```python
from build123d import *

# Parameters (mm, degrees)
SKETCH1_R           = 2.5
BOSS_EXTRUDE1_DEPTH = 6
SKETCH2_R           = 15
BOSS_EXTRUDE2_DEPTH = 2
BOSS_EXTRUDE3_START = 2
SKETCH3_R           = 15
BOSS_EXTRUDE3_DEPTH = 2
FILLET9_R           = 3
FILLET10_R          = 3
CUT_EXTRUDE1_DEPTH  = 10
SKETCH5_R           = 1.999371682
CUT_EXTRUDE2_DEPTH  = 0.7
SKETCH7_R           = 0.8
CUT_EXTRUDE6_DEPTH  = 3
SKETCH8_R           = 0.8
CUT_EXTRUDE7_DEPTH  = 5


with BuildPart() as part:
    # Sketch1 → Boss-Extrude1 (new body)
    with BuildSketch(Plane.XY):
        Circle(SKETCH1_R)
    extrude(amount=BOSS_EXTRUDE1_DEPTH)

    # Sketch2 → Boss-Extrude2 (add)
    with BuildSketch(Plane(origin=(0, 0, 0), x_dir=(-1, 0, 0), z_dir=(0, 0, -1))):
        Circle(SKETCH2_R)
    extrude(amount=BOSS_EXTRUDE2_DEPTH)

    # Sketch3 → Boss-Extrude3 (add)
    with BuildSketch(Plane.XY.offset(6).offset(BOSS_EXTRUDE3_START)):
        with Locations(Location((0, 0, 0), (0, 0, 180))):
            Circle(SKETCH3_R)
    extrude(amount=-BOSS_EXTRUDE3_DEPTH)

    # Fillet9
    fillet9_edges = [part.edges().sort_by_distance(p)[0] for p in [
        (-2.5, 0, 0),
    ]]
    fillet(fillet9_edges, radius=FILLET9_R)

    # Fillet10
    fillet10_edges = [part.edges().sort_by_distance(p)[0] for p in [
        (-2.5, 0, 6),
    ]]
    fillet(fillet10_edges, radius=FILLET10_R - 0.0001)  # a hair under: the kernel refuses the full size

    # Sketch4 → Cut-Extrude1 (cut)
    with BuildSketch(Plane(origin=(0, 0, -2), x_dir=(-1, 0, 0), z_dir=(0, 0, -1))):
        with BuildLine():
            Line((1.095333333, 1.096697264), (1.095333333, -1.096697264))
            ThreePointArc((1.095333333, -1.096697264), (-1.55, 0), (1.095333333, 1.096697264))
        make_face()
    extrude(amount=-CUT_EXTRUDE1_DEPTH, mode=Mode.SUBTRACT)

    # Sketch5 → Cut-Extrude2 (cut)
    with BuildSketch(Plane.XY.offset(8)):
        Circle(SKETCH5_R)
    extrude(amount=-CUT_EXTRUDE2_DEPTH, mode=Mode.SUBTRACT)

    # Sketch7 → Cut-Extrude6 (cut)
    with BuildSketch(Plane.XY.offset(8)):
        with Locations((4.509371682, 0)):
            Circle(SKETCH7_R)
        with Locations((-4.509371682, 0)):
            Circle(SKETCH7_R)
    extrude(amount=-CUT_EXTRUDE6_DEPTH, mode=Mode.SUBTRACT)

    # Sketch8 → Cut-Extrude7 (cut)
    with BuildSketch(Plane(origin=(0, 0, -2), x_dir=(-1, 0, 0), z_dir=(0, 0, -1))):
        with Locations((-4.5, 0)):
            Circle(SKETCH8_R)
        with Locations((4.5, 0)):
            Circle(SKETCH8_R)
    extrude(amount=-CUT_EXTRUDE7_DEPTH, mode=Mode.SUBTRACT)


solid = part.part
```
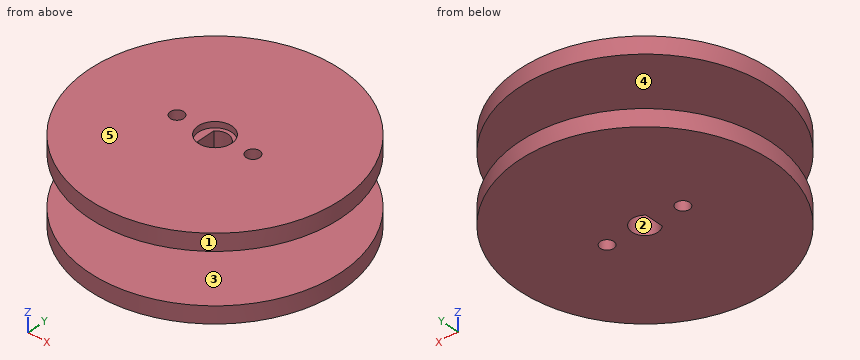
Geometry check sheet. Reference: the model listing, model coordinates, mm. Face numbers are marked on the shaded views. A direction names the side the tool comes from. Coordinates: 2 decimals unless noted, no trailing zeros. Order: outer loops, then holes, each group sorted by start corner. A loop starts at its lowest first (then second) coordinate and runs counter-clockwise, first axis right, second up. Notation, with made-up numbers: (61, 88) - (106, 88) arc R28 ccw to (106, 114) - close; hole circle Ø5 at (46.25, -19). An arc over 180 degrees is marked (long way). Answer as a JSON object with one key per item and string values. Group by question number.
Item 1: Scan lines: probe 1 along Z at (x, y) = (-8.5, 8); probe 2 along Y at (x, z) = (0, 7.5); probe 3 along Z at (x, y) = (-2, -4.25). Record each from-to range of solid material in increasing order.
Item 2: Tool access check on the marked faces 4 and 5. Record the directions out of +Z, -Z, +X, -X, +Y, -Y that give a thin tool (end or side, any length) a straight path to the whole face; none if there is none.
Item 3: Sectioned sample at C-C, the plane z = -1.25. Record the cut outline in (x, y).
Item 4: Depth check by flat-ended pin: pin 1 Ø6 at (x, z) = (-4, 5) entering from -Y; pin 2 Ø0.7 at (y, z) = (0, 4.5) entering from +X; pin 3 Ø4 at (x, z) = (8, 7) entering from -Y. Enter the tip coordinate at first touch or a pass-through.
Item 5: Sectioned sample at B-B, the plane y = -7. Record the cut outline in (x, z), and give its area (3 significant figures).
Item 6: Sectioned sample at A-A, the plane x = 8. Record the cut outline in (y, z).
Item 7: Draft check along Y on the marked faces 1, 2 and 3. Enter one of: +Y half, -Y half, draft (parallel to the pull), parting line (faces both ways), or undercut.
Resolved:
{
 "1": {"probe 1": "-2 to 0, 6 to 8", "probe 2": "-15 to -2, 2 to 15", "probe 3": "-2 to 0.11, 5.89 to 8"},
 "2": {"face 4": "none", "face 5": "+Z, +X, -X, +Y, -Y"},
 "3": {"outline": "circle Ø30 at (0, 0); hole circle Ø1.6 at (-4.5, 0); hole (-1.1, -1.1) arc R1.55 ccw (long way) to (-1.1, 1.1) - close; hole circle Ø1.6 at (4.5, 0)"},
 "4": {"pin 1": "y = -14.95", "pin 2": "x = 3.14", "pin 3": "y = -13.75"},
 "5": {"outline": "(-13.27, -2) - (13.27, -2) - (13.27, 0) - (-13.27, 0) - close; (-13.27, 6) - (13.27, 6) - (13.27, 8) - (-13.27, 8) - close", "area": "106 mm^2"},
 "6": {"outline": "(-12.69, -2) - (12.69, -2) - (12.69, 0) - (-12.69, 0) - close; (-12.69, 6) - (12.69, 6) - (12.69, 8) - (-12.69, 8) - close"},
 "7": {"face 1": "parting line", "face 2": "undercut", "face 3": "draft"}
}
